Verification items for the finished model (mm, model axes). Face numbers are marked on the shaded views. A direction names the side the tool comes from. Give positions to 0.01 mm unless a question says otherwise; leave off trailing zeros. Loops run counter-clockwise (first coordinate to the right, second up) from the corner with the lowest first, then second, coordinate; pieces in that order, holes last. Notation, with made-up numbers: (-28.75, 61.25) - (-15.75, 61.25) arc R23 ccw to (-15.75, 90.25) - close; hole circle Ø8 at (9, 33). An arc over 180 degrees is marked (long way). One line per question, with ' | ' between items. Start each with the question number.
1. Depth check by flat-ended pin: pin 1 Ø9 at (x, y) = (12.5, -3.5) entering from -Z; pin 2 Ø3.5 at (x, y) = (7.5, -9) entering from -Z. Enter the tip coordinate at first touch or a pass-through.
2. Thickness scan on line 1 along Y through (x, z) = (17.5, 3.4); line 2 along X through (y, z) = (-16, 6.5); line 3 along Z through (x, y) = (-12, -25). Record the ranges inside material, lowest first. Write a range as from..to.
3. Section check D-D, the plane z = 1. Enter the section's corners in (x, y), then the cut area to 3 significant figures.
4. Tool access check on the marked faces 1 and 2. Record the directions out of +Z, -Z, +X, -X, +Y, -Y that give a thin tool (end or side, any length) a straight path to the whole face; none if there is none.
5. Section check B-B, the plane x = -12. Enter the section's corners in (y, z), then the cut area to 3 significant figures.
6. Section check C-C, the plane y = -14. Enter the section's corners in (x, z).
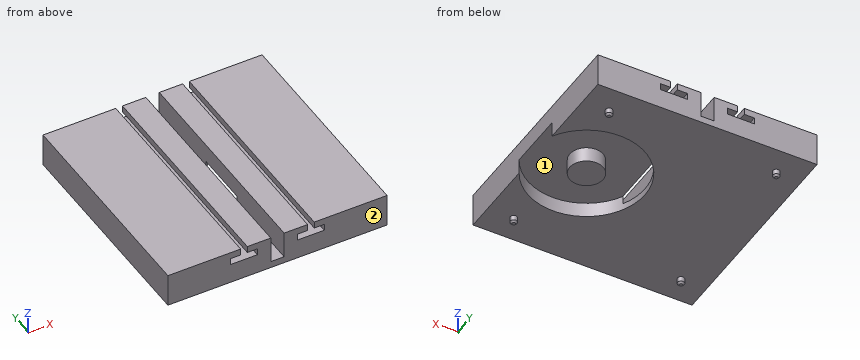
from build123d import *

# Parameters (mm, degrees)
SKETCH_W        = 65.5
SKETCH_H        = 65.5
PAD_DEPTH       = 10
POCKET_DEPTH    = 65.501
SKETCH002_W     = 4
SKETCH002_H     = 65.5
POCKET001_DEPTH = 8
SKETCH003_R     = 17.5
POCKET002_DEPTH = 4.5
SKETCH004_R     = 5
PAD001_DEPTH    = 4.5
SKETCH005_R     = 1
PAD002_DEPTH    = 2
CHAMFER_SIZE    = 0.5


with BuildPart() as part:
    # Sketch → Pad (new body)
    with BuildSketch(Plane.XY):
        Rectangle(SKETCH_W, SKETCH_H)
    extrude(amount=PAD_DEPTH)

    # Sketch001 (on Face3 of Pad) → Pocket (cut, through all)
    with BuildSketch(Plane.XZ.offset(32.75)):
        Polygon((-11.000005, 10), (-11.000005, 8), (-14.000005, 8), (-14.000005, 6), (-6.000005, 6), (-6.000005, 8), (-9.000005, 8), (-8.999995, 10), align=None)
        Polygon((8.999995, 10), (8.999995, 8), (5.999995, 8), (5.999995, 6), (13.999995, 6), (13.999995, 8), (10.999995, 8), (10.999995, 10), align=None)
    extrude(amount=-POCKET_DEPTH, mode=Mode.SUBTRACT)

    # Sketch002 (on Face12 of Pocket) → Pocket001 (cut)
    with BuildSketch(Plane.XY.offset(10)):
        Rectangle(SKETCH002_W, SKETCH002_H)
    extrude(amount=-POCKET001_DEPTH, mode=Mode.SUBTRACT)

    # Sketch003 (on Face2 of Pocket001) → Pocket002 (cut)
    with BuildSketch(Plane(origin=(0, 0, 0), x_dir=(1, 0, 0), z_dir=(0, 0, -1))):
        with Locations((17.5, 0)):
            Circle(SKETCH003_R)
    extrude(amount=-POCKET002_DEPTH, mode=Mode.SUBTRACT)

    # Sketch004 (on Face28 of Pocket002) → Pad001 (join)
    with BuildSketch(Plane(origin=(0, 0, 4.5), x_dir=(1, 0, 0), z_dir=(0, 0, -1))):
        with Locations((17.5, 0)):
            Circle(SKETCH004_R)
    extrude(amount=PAD001_DEPTH)

    # Sketch005 (on Face2 of Pad001) → Pad002 (join)
    with BuildSketch(Plane(origin=(0, 0, 0), x_dir=(1, 0, 0), z_dir=(0, 0, -1))):
        with Locations((-25, 25)):
            Circle(SKETCH005_R)
        with Locations((25, 25)):
            Circle(SKETCH005_R)
        with Locations((-25, -25)):
            Circle(SKETCH005_R)
        with Locations((25, -25)):
            Circle(SKETCH005_R)
    extrude(amount=PAD002_DEPTH)

    # Chamfer
    chamfer_edges = [part.edges().sort_by_distance(p)[0] for p in [
        (-26, -25, -2),
        (-26, 25, -2),
        (24, 25, -2),
        (24, -25, -2),
    ]]
    chamfer(chamfer_edges, length=CHAMFER_SIZE)


solid = part.part
Results list:
1) pin 1: z = 0 | pin 2: z = 4.5
2) line 1: -32.75..-17.5, -5..5, 17.5..32.75 | line 2: -32.75..-14, -6..-2, 2..6, 14..32.75 | line 3: 0..6, 8..10
3) outline: (-32.75, -32.75) - (32.75, -32.75) - (32.75, -8.58) arc R17.5 cw (long way) to (32.75, 8.58) - (32.75, 32.75) - (-32.75, 32.75) - close; circle Ø10 at (17.5, 0) | area: 3,430 mm²
4) face 1: -Z | face 2: +Z, -Z, +X, -X, -Y
5) outline: (-32.75, 0) - (32.75, 0) - (32.75, 6) - (-32.75, 6) - close; (-32.75, 8) - (32.75, 8) - (32.75, 10) - (-32.75, 10) - close | area: 524 mm²
6) outline: (-32.75, 0) - (7, 0) - (7, 4.5) - (28, 4.5) - (28, 0) - (32.75, 0) - (32.75, 10) - (11, 10) - (11, 8) - (14, 8) - (14, 6) - (6, 6) - (6, 8) - (9, 8) - (9, 10) - (2, 10) - (2, 2) - (-2, 2) - (-2, 10) - (-9, 10) - (-9, 8) - (-6, 8) - (-6, 6) - (-14, 6) - (-14, 8) - (-11, 8) - (-11, 10) - (-32.75, 10) - close
